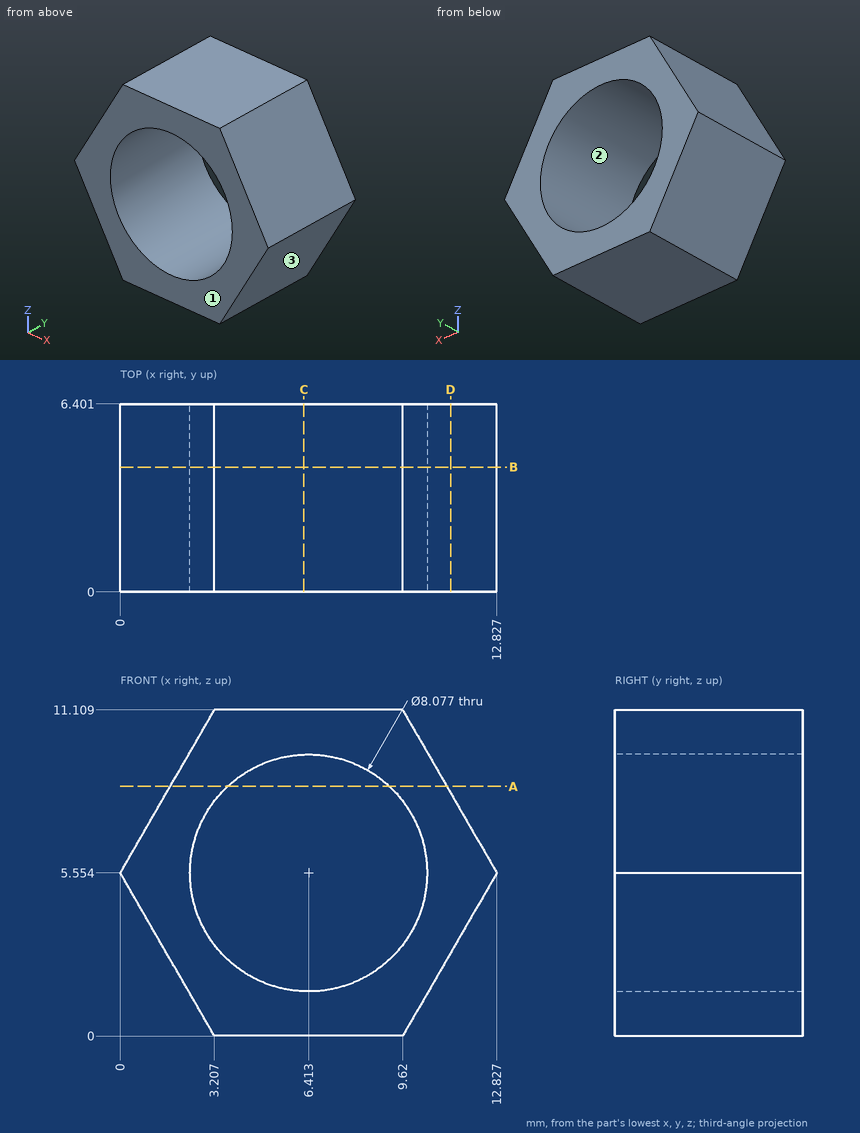
Check sheet for the drawn part. Datum: minimum x, y, z corner. Units: mm. Give positions to 0.01 mm unless a question says otherwise; leave off trailing zeros. Write each loop counter-clockwise with the first axis right and the second up, starting at its lowest first coordinate (ties: lowest second). Pieces come first, ordered by that corner, then holes. Notation, with made-up numbers: (59.5, 26.25) -> (109.5, 26.25) arc R24 ccw to (109.5, 38.25) -> close; hole circle Ø6 at (43.5, 27.5). An arc over 180 degrees is marked (long way). Use one line per item in the form item = value. Start each with the question number.
1. Section check D-D (x = 11.25). Record the cut outline in (y, z) (1 decimal).
2. Go/stop test with flat-tipped pins: P1, Ø3, axis at x = 7.5, z = 6.5, coming from the +Y side; P2, Ø1.5, axis at y = 1, z = 3, coming from the -X side. Record where each tip stops, or that it passes through.
3. Section check C-C (x = 6.25). Record the cut outline in (y, z).
4. Thickness scan on line 1 along X through (y, z) = (6, 9) (1 decimal); line 2 along Z through (x, y) = (3.75, 4.25); line 3 along Z through (x, y) = (8.5, 1.25) (1 decimal). Record the ranges inside material, lowest first. Write a range as from..to.
5. Mould release check, pull along X, two halves, no side actions. Record for the marked faces 1, 2 and 3: pulls with the +X half, pulls with the -X half, needs draft (parallel to the pull), parting line crosses it, or undercut.
6. Section check B-B (y = 4.25). Record the cut outline in (x, z) (1 decimal).
7. Section check A-A (z = 8.5). Record the cut outline in (x, y).
Conclusion:
q1.outline = (0, 2.8) -> (6.4, 2.8) -> (6.4, 8.3) -> (0, 8.3) -> close
q2.P1 = through
q2.P2 = 1.04
q3.outline = (0, 0) -> (6.4, 0) -> (6.4, 1.52) -> (0, 1.52) -> close; (0, 9.59) -> (6.4, 9.59) -> (6.4, 11.11) -> (0, 11.11) -> close
q4.line_1 = 2..4.3, 8.5..10.8
q4.line_2 = 0..2.52, 8.59..11.11
q4.line_3 = 0..2.1, 9..11.1
q5.face_1 = needs draft
q5.face_2 = undercut
q5.face_3 = pulls with the +X half
q6.outline = (0, 5.6) -> (3.2, 0) -> (9.6, 0) -> (12.8, 5.6) -> (9.6, 11.1) -> (3.2, 11.1) -> close; hole circle Ø8.1 at (6.4, 5.6)
q7.outline = (1.7, 0) -> (3.65, 0) -> (3.65, 6.4) -> (1.7, 6.4) -> close; (9.18, 0) -> (11.13, 0) -> (11.13, 6.4) -> (9.18, 6.4) -> close
